```python
from build123d import *

# Parameters (mm, degrees)
SKETCH1_R           = 20
BOSS_EXTRUDE1_DEPTH = 2
SKETCH2_R           = 4
BOSS_EXTRUDE2_DEPTH = 12
CUT_EXTRUDE1_REACH  = 34.496
SKETCH3_R           = 2.525
CHAMFER2_SIZE       = 1


with BuildPart() as part:
    # Sketch1 → Boss-Extrude1 (new, symmetric)
    with BuildSketch(Plane.XY):
        Circle(SKETCH1_R)
    extrude(amount=BOSS_EXTRUDE1_DEPTH, both=True)

    # Sketch2 → Boss-Extrude2 (add)
    with BuildSketch(Plane.XY.offset(2)):
        with Locations((12, 0)):
            Circle(SKETCH2_R)
    extrude(amount=BOSS_EXTRUDE2_DEPTH)

    # Sketch3 → Cut-Extrude1 (cut, up to next)
    with BuildSketch(Plane(origin=(0, 0, -2), x_dir=(-1, 0, 0), z_dir=(0, 0, -1)), mode=Mode.PRIVATE) as cut_extrude1_sk1:
        Circle(SKETCH3_R)
    cut_extrude1_tool1 = extrude(cut_extrude1_sk1.sketch, amount=-CUT_EXTRUDE1_REACH, mode=Mode.PRIVATE) & part.part
    add(cut_extrude1_tool1.solids().sort_by_distance((0, 0, -2))[0], mode=Mode.SUBTRACT)

    # Chamfer2
    chamfer2_edges = [part.edges().sort_by_distance(p)[0] for p in [
        (-20, 0, -2),
        (-20, 0, 2),
        (8, 0, 14),
    ]]
    chamfer(chamfer2_edges, length=CHAMFER2_SIZE)


solid = part.part
```
Source: CAD feature listing. Evaluate the final solid. Frame: model axes, mm. A direction names the side the tool comes from. Coordinates: 2 decimals unless noted, no trailing zeros. Loops run counter-clockwise (first coordinate to the right, second up) from the corner with the lowest first, then second, coordinate; pieces in that order, holes last. Notation, with made-up numbers: (41, 69) -> (55, 69) arc R5 ccw to (55, 75) -> close; hole circle Ø5 at (63, -13.75). An arc over 180 degrees is marked (long way). One line per item, written item: value. Start each with the question number.
Q1. Section query C-C, the plane z = 0. Return the cut outline in (x, y) (3 decimals), and give its area (3 significant figures).
Q2. Contact query for flat-ended pins moving along their axis: P1, Ø4, axis at y = 12, z = 0, coming from the +X side; P2, Ø1.5, axis at x = 12, z = 1, coming from the +Y side; P3, Ø3, axis at x = 13, z = 6, coming from the +Y side. Output: stop coordinate, or through.
Q3. Set-up query: faces 4 (the face through (0, -4, -2)), 5 (the face through (8.8, -2.4, 7.4)). Return all of +Z, -Z, +X, -X, +Y, -Y with unobstructed straight access to the full face (end or side cutting, diameter ignored); none if empty.
Q4. Line query: line 1 along Y through (x, z) = (0, 0.15) (3 decimals); line 2 along Z through (x, y) = (15, -7); line 3 along X through (y, z) = (14, 0). Output: solid intervals per line, ascending.
Q5. Mould query, pull axis Y, two halves, no side actions, for faces 1 (the face through (-4.336, -19.524, 0.014)), 2 (the face through (-2.41, 0.76, -0.03)), 3 (the face through (12, 0, 14)). Classes: pulls with the +Y half, pulls with the -Y half, needs draft (parallel to the pull), parting line crosses it, or undercut.
Q6. Section query D-D, the plane z = 6. Return the cut outline in (x, y), and give its area (3 significant figures).
Q7. Section query B-B, the plane y = 0. Return the cut outline in (x, z) (3 decimals).
Q8. Section query A-A, the plane x = 0. Return the cut outline in (y, z) (3 decimals).
Results:
1. outline: circle Ø40 at (0, 0); hole circle Ø5.05 at (0, 0)
1. area: 1,240 mm^2
2. P1: x = 17.32
2. P2: y = 16.54
2. P3: y = 4
3. face 4: -Z, +X, -X, +Y, -Y
3. face 5: +Z
4. line 1: -20 to -2.525, 2.525 to 20
4. line 2: -2 to 2
4. line 3: -14.28 to 14.28
5. face 1: parting line crosses it
5. face 2: undercut
5. face 3: needs draft
6. outline: circle Ø8 at (12, 0)
6. area: 50.3 mm^2
7. outline: (-20, -1) -> (-19, -2) -> (-2.525, -2) -> (-2.525, 2) -> (-19, 2) -> (-20, 1) -> close; (2.525, -2) -> (19, -2) -> (20, -1) -> (20, 1) -> (19, 2) -> (16, 2) -> (16, 13) -> (15, 14) -> (9, 14) -> (8, 13) -> (8, 2) -> (2.525, 2) -> close
8. outline: (-20, -1) -> (-19, -2) -> (-2.525, -2) -> (-2.525, 2) -> (-19, 2) -> (-20, 1) -> close; (2.525, -2) -> (19, -2) -> (20, -1) -> (20, 1) -> (19, 2) -> (2.525, 2) -> close
